For this review, take the finished solid that the model builds, in its own axes (mm). Round coordinates to 2 decimals unless told otherwise and drop trailing zeros. Order: outer loops, then holes, each group sorted by start corner. A loop starts at its lowest first (then second) coordinate and runs counter-clockwise, first axis right, second up. Notation, with made-up numbers: M 47.25,59.25 L 79.25,59.25 A22 cw 79.25,66.25 Z; hole C 72,-20.75 d8. An arc over 180 degrees is marked long. Put each result on its own line as item: value.
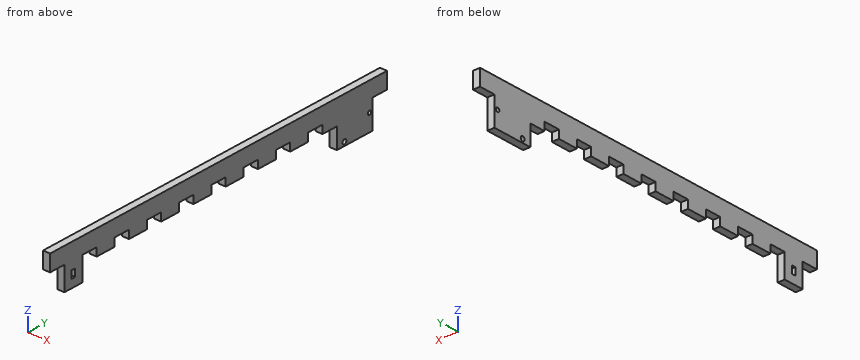
from build123d import *

# Parameters (mm, degrees)
BOSS_EXTRUDE1_DEPTH = 5.588
SKETCH2_W           = 22.3499934
SKETCH2_H           = 31.75
SKETCH2_R           = 1.55
SKETCH2_R_2         = 1.7
BOSS_EXTRUDE2_DEPTH = 5.588


with BuildPart() as part:
    # Sketch1 → Boss-Extrude1 (new body)
    with BuildSketch(Plane(origin=(0, 0, 0), x_dir=(0, 0, -1), z_dir=(1, 0, 0))):
        Polygon((3.175, 120.65), (9.525, 120.65), (9.525, 136.525), (3.175, 136.525), (3.175, 149.225), (-9.525, 149.225), (-9.525, -149.225), (3.175, -149.225), (3.175, -136.525), (9.525, -136.525), (9.525, -120.65), (3.175, -120.65), (3.175, -107.95), (9.525, -107.95), (9.525, -92.075), (3.175, -92.075), (3.175, -79.375), (9.525, -79.375), (9.525, -63.5), (3.175, -63.5), (3.175, -50.8), (9.525, -50.8), (9.525, -34.925), (3.175, -34.925), (3.175, -22.225), (9.525, -22.225), (9.525, -6.35), (3.175, -6.35), (3.175, 6.35), (9.525, 6.35), (9.525, 22.225), (3.175, 22.225), (3.175, 34.925), (9.525, 34.925), (9.525, 50.8), (3.175, 50.8), (3.175, 63.5), (9.525, 63.5), (9.525, 79.375), (3.175, 79.375), (3.175, 92.075), (9.525, 92.075), (9.525, 107.95), (3.175, 107.95), align=None)
    extrude(amount=BOSS_EXTRUDE1_DEPTH)

    # Sketch2 → Boss-Extrude2 (add)
    with BuildSketch(Plane(origin=(5.588, 0, 0), x_dir=(0, 0, -1), z_dir=(1, 0, 0))):
        Polygon((21.717, -120.65), (9.525, -120.65), (9.525, -127), (15.367, -127), (15.367, -130.175), (9.525, -130.175), (9.525, -136.525), (21.717, -136.525), align=None)
        with Locations((14.3499967, 120.65)):
            Rectangle(SKETCH2_W, SKETCH2_H)
        with Locations((12.3249992, 133.7250056)):
            Circle(SKETCH2_R, mode=Mode.SUBTRACT)
        with Locations((22.6249992, 111.5250056)):
            Circle(SKETCH2_R_2, mode=Mode.SUBTRACT)
    extrude(amount=-BOSS_EXTRUDE2_DEPTH)


solid = part.part
(1) To check wall thickness, follow L1, parallel to Y at x = 3.3, z = -12.5 (3 decimals); L2, parallel to Y at x = 1.05, z = -16 (3 decimals); L3, parallel to Y at x = 1.45, z = -22.5 (3 decimals). State the ranges of each line that lie inside material, in increasing order.
A:
L1: y = -136.525 to -130.175, -127 to -120.65, 104.775 to 132.185, 135.265 to 136.525
L2: y = -136.525 to -120.65, 104.775 to 136.525
L3: y = 104.775 to 109.83, 113.22 to 136.525
(2) Add section A-A on z = -7. State how many separate pieces and enclosed holes the cut face has, then the cut area to 3 significant figures.
A:
separate pieces: 9
enclosed holes: 0
area: 958 mm2
(3) Add section D-D on y = 57.5. Give the boundary of the cut face in (x, z) (3 decimals), then the cut area to 3 significant figures.
A:
outline: M 0,-3.175 L 5.588,-3.175 L 5.588,9.525 L 0,9.525 Z
area: 71.0 mm2
(4) Insertion check: pin 1 Ø3 at (x, y) = (1.5, -51) entering from -Z (3 decimals); pin 2 Ø3 at (x, z) = (2.5, -6.5) entering from +Y (3 decimals); pin 3 Ø1 at (x, y) = (2.5, -128) entering from -Z. Each pin has a flat end and moves straight along its axis. Give the tip position at first contact, or say it passes through.
A:
pin 1: stops at z = -9.525
pin 2: stops at y = 136.525
pin 3: stops at z = -21.72
(5) Add section B-B on y = 97. Give the boundary of the cut face in (x, z) (3 decimals).
A:
outline: M 0,-9.525 L 5.588,-9.525 L 5.588,9.525 L 0,9.525 Z
